```python
from build123d import *

# Parameters (mm, degrees)
BOSS_EXTRUDE1_DEPTH = 5
SKETCH2_W           = 55
SKETCH2_H           = 13
SKETCH2_R           = 3
BOSS_EXTRUDE2_DEPTH = 11.5
SKETCH3_W           = 11.5
SKETCH3_H           = 13
BOSS_EXTRUDE3_DEPTH = 55
BOSS_EXTRUDE4_DEPTH = 60
CUT_EXTRUDE1_DEPTH  = 35
SKETCH6_R           = 2.5
SKETCH6_R_2         = 2
CUT_EXTRUDE2_DEPTH  = 10
SKETCH7_R           = 2.6
CUT_EXTRUDE3_DEPTH  = 10
SKETCH8_R           = 3
CUT_EXTRUDE4_DEPTH  = 6
FILLET1_R           = 10
FILLET2_R           = 3
FILLET3_R           = 10


with BuildPart() as part:
    # Sketch1 → Boss-Extrude1 (new body)
    with BuildSketch(Plane(origin=(0, 0, 0), x_dir=(1, 0, 0), z_dir=(0, 1, 0))):
        Polygon((130, 85), (90, 85), (90, 25), (110, 25), (110, -55), (-88, -55), (-88, -27), (-110, -27), (-110, 85), (-130, 85), (-130, -85), (130, -85), align=None)
    extrude(amount=BOSS_EXTRUDE1_DEPTH)

    # Sketch2 → Boss-Extrude2 (add)
    with BuildSketch(Plane(origin=(0, 5, 0), x_dir=(1, 0, 0), z_dir=(0, 1, 0))):
        with Locations((102.5, -61.5)):
            Rectangle(SKETCH2_W, SKETCH2_H)
        with Locations(Location((81.5, -61.5, 0), (0, 0, 270))):
            Circle(SKETCH2_R, mode=Mode.SUBTRACT)
        with Locations(Location((123.5, -61.5, 0), (0, 0, 270))):
            Circle(SKETCH2_R, mode=Mode.SUBTRACT)
    extrude(amount=BOSS_EXTRUDE2_DEPTH)

    # Sketch3 → Boss-Extrude3 (add)
    with BuildSketch(Plane(origin=(0, 5, 0), x_dir=(1, 0, 0), z_dir=(0, 1, 0))):
        with Locations((124.25, 31.5)):
            Rectangle(SKETCH3_W, SKETCH3_H)
    extrude(amount=BOSS_EXTRUDE3_DEPTH)

    # Sketch4 → Boss-Extrude4 (add)
    with BuildSketch(Plane(origin=(0, 0, -85), x_dir=(-1, 0, 0), z_dir=(0, 0, -1))):
        with BuildLine():
            Line((-90, 5), (-83.30854382, 5))
            ThreePointArc((-83.30854382, 5), (-70.704531681, -10.206792987), (-51.737752976, -4.695987191))
            Line((-51.737752976, -4.695987191), (-43.449337938, 5))
            Line((-43.449337938, 5), (110, 5))
            Line((110, 5), (130, 5))
            Line((130, 5), (130, 0))
            Line((130, 0), (110, 0))
            Line((110, 0), (-41.80340478, 0))
            Line((-41.80340478, 0), (-48.31719122, -7.619983989))
            ThreePointArc((-48.31719122, -7.619983989), (-69.790001662, -15.071544701), (-86.80340478, 0))
            Line((-86.80340478, 0), (-90, 0))
            Line((-90, 0), (-130, 0))
            Line((-130, 0), (-130, 5))
            Line((-130, 5), (-90, 5))
        make_face()
    extrude(amount=-BOSS_EXTRUDE4_DEPTH)

    # Sketch5 → Cut-Extrude1 (cut)
    with BuildSketch(Plane(origin=(0, 0, -85), x_dir=(-1, 0, 0), z_dir=(0, 0, -1))):
        with BuildLine():
            Line((130, 5), (130, 0))
            Line((130, 0), (-41.80340478, 0))
            Line((-41.80340478, 0), (-48.31719122, -7.619983989))
            ThreePointArc((-48.31719122, -7.619983989), (-69.790001662, -15.071544701), (-86.80340478, 0))
            Line((-86.80340478, 0), (-130, 0))
            Line((-130, 0), (-130, 5))
            Line((-130, 5), (-83.30854382, 5))
            ThreePointArc((-83.30854382, 5), (-70.704531681, -10.206792987), (-51.737752976, -4.695987191))
            Line((-51.737752976, -4.695987191), (-43.449337938, 5))
            Line((-43.449337938, 5), (130, 5))
        make_face()
    extrude(amount=-CUT_EXTRUDE1_DEPTH, mode=Mode.SUBTRACT)

    # Sketch6 → Cut-Extrude2 (cut)
    with BuildSketch(Plane(origin=(0, 5, 0), x_dir=(1, 0, 0), z_dir=(0, 1, 0))):
        with Locations(Location((-104, -31, 0), (0, 0, 270))):
            Circle(SKETCH6_R)
        with Locations(Location((-92, -31, 0), (0, 0, 270))):
            Circle(SKETCH6_R)
        with Locations(Location((-92, -43, 0), (0, 0, 270))):
            Circle(SKETCH6_R)
        with Locations(Location((-104, -43, 0), (0, 0, 270))):
            Circle(SKETCH6_R)
        with Locations(Location((-9.17, -59, 0), (0, 0, 270))):
            Circle(SKETCH6_R_2)
        with Locations(Location((-69.17, -59, 0), (0, 0, 270))):
            Circle(SKETCH6_R_2)
    extrude(amount=-CUT_EXTRUDE2_DEPTH, mode=Mode.SUBTRACT)

    # Sketch7 → Cut-Extrude3 (cut)
    with BuildSketch(Plane(origin=(0, 5, 0), x_dir=(1, 0, 0), z_dir=(0, 1, 0))):
        with Locations(Location((120, 15.5, 0), (0, 0, 270))):
            Circle(SKETCH7_R)
        with Locations(Location((120, -50.5, 0), (0, 0, 270))):
            Circle(SKETCH7_R)
        with Locations(Location((-120, -50.5, 0), (0, 0, 270))):
            Circle(SKETCH7_R)
        with Locations(Location((-120, 15.5, 0), (0, 0, 270))):
            Circle(SKETCH7_R)
    extrude(amount=-CUT_EXTRUDE3_DEPTH, mode=Mode.SUBTRACT)

    # Sketch8 → Cut-Extrude4 (cut)
    with BuildSketch(Plane.ZY.offset(-118.5)):
        with Locations((-31.5, 53.5)):
            Circle(SKETCH8_R)
        with Locations((-31.5, 11.5)):
            Circle(SKETCH8_R)
    extrude(amount=-CUT_EXTRUDE4_DEPTH, mode=Mode.SUBTRACT)

    # Fillet1
    fillet1_edges = [part.edges().sort_by_distance(p)[0] for p in [
        (75, 5, 61.5),
        (102.5, 5, 68),
        (124.25, 5, -38),
    ]]
    fillet(fillet1_edges, radius=FILLET1_R)

    # Fillet2
    fillet2_edges = [part.edges().sort_by_distance(p)[0] for p in [
        (124.25, 5, -25),
    ]]
    fillet(fillet2_edges, radius=FILLET2_R)

    # Fillet3
    fillet3_edges = [part.edges().sort_by_distance(p)[0] for p in [
        (86.80340478, 0, -37.5),
        (41.80340478, 0, -37.5),
    ]]
    fillet(fillet3_edges, radius=FILLET3_R)


solid = part.part
```
Model file for the job. Use its own axes, mm. A direction names the side the tool comes from. Coordinates: 2 decimals unless noted, no trailing zeros. Loops run counter-clockwise (first coordinate to the right, second up) from the corner with the lowest first, then second, coordinate; pieces in that order, holes last. Notation, with made-up numbers: (84.25, 31.25) - (94.25, 31.25) arc R21 cw to (94.25, 37.25) - close; hole circle Ø2 at (10, -16.75). An arc over 180 degrees is marked (long way). Write item = value, one per line. Start each with the question number.
Item 1: Pull direction Z, two halves, no side cores. Call faces 4 (the face through (-89.52, 2.53, 30.67)), 5 (the face through (124.33, 7.85, -41.01)), 6 (the face through (71.99, 7.85, 63.78)): +Z half, -Z half, draft (parallel to the pull), parting line (faces both ways), or undercut.
Item 2: Saw through at D-D, the plane x = 62.5. List the corners of the cut face in (y, z), then the cut area to 3 significant figures.
Item 3: Saw through at C-C, the plane z = -15.5. List the corners of the cut face in (x, y).
Item 4: Saw through at A-A, the plane z = 15. List the corners of the cut face in (x, y), then the cut area to 3 significant figures.
Item 5: 3-axis set-ups, long thin cutter, end or side, ignore diameter. For faces 1 (the face through (44, 4, 55)), 2 (the face through (112, 5, -10)), 3 (the face through (-1, 1, -25)): which of +Z, -Z, +X, -X, +Y, -Y reach the whole face in a straight line?
Item 6: Saw through at B-B, the plane x = -104. List the corners of the cut face in (y, z), then the cut area to 3 significant figures.
Item 7: Drop flat-ended pins along their axis: pin 1 Ø8 at (x, z) = (12, 60.5) entering from +Y; pin 2 Ø7 at (x, z) = (123.5, 61.5) entering from +Y; pin 3 Ø7 at (x, z) = (-120, -15.5) entering from -Y; pin 4 Ø13 at (x, y) = (-1, 6.5) entering from -Z. Give the stop position or say it passes through.
Item 8: Wall check: probe 1 along X at (y, z) = (1.6, 31); probe 2 along X at (y, z) = (3, 50); probe 3 along X at (y, z) = (1, 59). Give the ranges that are in metal, low to high. Write a range as [from, to].
Answers:
q1.face_4 = undercut
q1.face_5 = -Z half
q1.face_6 = draft
q2.outline = (-15.31, -50) - (-10.76, -50) - (-10.76, -25) - (-15.31, -25) - close; (0, 55) - (5, 55) - (5, 85) - (0, 85) - close
q2.area = 264 mm2
q3.outline = (-130, 0) - (-122.6, 0) - (-122.6, 5) - (-130, 5) - close; (-117.4, 0) - (-110, 0) - (-110, 5) - (-117.4, 5) - close; (110, 0) - (117.4, 0) - (117.4, 5) - (110, 5) - close; (122.6, 0) - (130, 0) - (130, 5) - (122.6, 5) - close
q4.outline = (-130, 0) - (-110, 0) - (-110, 5) - (-130, 5) - close; (110, 0) - (130, 0) - (130, 5) - (110, 5) - close
q4.area = 200 mm2
q5.face_1 = +Y
q5.face_2 = -X, +Y
q5.face_3 = +Y, -Y
q6.outline = (0, -50) - (5, -50) - (5, -25) - (0, -25) - close; (0, 27) - (5, 27) - (5, 28.5) - (0, 28.5) - close; (0, 33.5) - (5, 33.5) - (5, 40.5) - (0, 40.5) - close; (0, 45.5) - (5, 45.5) - (5, 85) - (0, 85) - close
q6.area = 365 mm2
q7.pin_1 = 5
q7.pin_2 = 16.5
q7.pin_3 = 0
q7.pin_4 = -50
q8.probe_1 = [-130, -106.5], [-101.5, -94.5], [-89.5, -88], [110, 130]
q8.probe_2 = [-130, -122.55], [-117.45, -88], [110, 117.45], [122.55, 130]
q8.probe_3 = [-130, -71.17], [-67.17, -11.17], [-7.17, 130]
